```python
from build123d import *

# Parameters (mm, degrees)
SKETCH_1_R      = 1.5
EXTRUDE_1_DEPTH = 5
EXTRUDE_2_DEPTH = 10
FILLET_1_R      = 2
SKETCH_4_R      = 4.5
EXTRUDE_4_DEPTH = 110


with BuildPart() as part:
    # 草图1 → 凸台-拉伸1 (new body)
    with BuildSketch(Plane(origin=(0, 0, 0), x_dir=(1, 0, 0), z_dir=(0, 1, 0))):
        with BuildLine():
            Line((-65.462788351, 64.203800201), (-65.462788351, -59.796199799))
            ThreePointArc((-65.462788351, -59.796199799), (-64.584108695, -61.917520143), (-62.462788351, -62.796199799))
            Line((-62.462788351, -62.796199799), (158.823574937, -62.796199799))
            ThreePointArc((158.823574937, -62.796199799), (160.944895281, -61.917520143), (161.823574937, -59.796199799))
            Line((161.823574937, -59.796199799), (161.823574937, 64.203800201))
            ThreePointArc((161.823574937, 64.203800201), (160.944895281, 66.325120544), (158.823574937, 67.203800201))
            Line((158.823574937, 67.203800201), (-62.462788351, 67.203800201))
            ThreePointArc((-62.462788351, 67.203800201), (-64.584108695, 66.325120544), (-65.462788351, 64.203800201))
        make_face()
        with Locations(Location((-11.819606707, -57.796199799, 0), (0, 0, 270))):
            Circle(SKETCH_1_R, mode=Mode.SUBTRACT)
        with Locations(Location((108.180393293, -57.796199799, 0), (0, 0, 90))):
            Circle(SKETCH_1_R, mode=Mode.SUBTRACT)
        with Locations(Location((108.180393293, 62.203800201, 0), (0, 0, 270))):
            Circle(SKETCH_1_R, mode=Mode.SUBTRACT)
        with Locations(Location((-11.819606707, 62.203800201, 0), (0, 0, 90))):
            Circle(SKETCH_1_R, mode=Mode.SUBTRACT)
    extrude(amount=EXTRUDE_1_DEPTH)

    # 草图2 → 凸台-拉伸2 (add)
    with BuildSketch(Plane(origin=(0, 5, 0), x_dir=(1, 0, 0), z_dir=(0, 1, 0))):
        with BuildLine():
            Line((48.180393293, -62.796199799), (158.823574937, -62.796199799))
            ThreePointArc((158.823574937, -62.796199799), (160.944895281, -61.917520143), (161.823574937, -59.796199799))
            Line((161.823574937, -59.796199799), (161.823574937, 64.203800201))
            ThreePointArc((161.823574937, 64.203800201), (160.944895281, 66.325120544), (158.823574937, 67.203800201))
            Line((158.823574937, 67.203800201), (-62.462788351, 67.203800201))
            ThreePointArc((-62.462788351, 67.203800201), (-64.584108695, 66.325120544), (-65.462788351, 64.203800201))
            Line((-65.462788351, 64.203800201), (-65.462788351, -59.796199799))
            ThreePointArc((-65.462788351, -59.796199799), (-64.584108695, -61.917520143), (-62.462788351, -62.796199799))
            Line((-62.462788351, -62.796199799), (48.180393293, -62.796199799))
        make_face()
        Polygon((48.180393293, -52.796199799), (151.823574937, -52.796199799), (151.823574937, 57.203800201), (-55.462788351, 57.203800201), (-55.462788351, -52.796199799), align=None, mode=Mode.SUBTRACT)
    extrude(amount=EXTRUDE_2_DEPTH)

    # 圆角1
    fillet_1_edges = [part.edges().sort_by_distance(p)[0] for p in [
        (48.180393293, 15, 62.796199799),
        (160.944895281, 15, 61.917520143),
        (161.823574937, 15, -2.203800201),
        (160.944895281, 15, -66.325120544),
        (48.180393293, 15, -67.203800201),
        (-64.584108695, 15, -66.325120544),
        (-65.462788351, 15, -2.203800201),
        (-64.584108695, 15, 61.917520143),
    ]]
    fillet(fillet_1_edges, radius=FILLET_1_R)

    # 草图4 → 凸台-拉伸4 (add)
    with BuildSketch(Plane(origin=(0, 0, 52.796199799), x_dir=(-1, 0, 0), z_dir=(0, 0, -1))):
        with Locations(Location((-146.823574937, 12, 0), (0, 0, 138.189685104))):
            Circle(SKETCH_4_R)
        with Locations(Location((-136.973574937, 12, 0), (0, 0, 138.189685104))):
            Circle(SKETCH_4_R)
        with Locations(Location((-127.123574937, 12, 0), (0, 0, 138.189685104))):
            Circle(SKETCH_4_R)
        with Locations(Location((-117.273574937, 12, 0), (0, 0, 138.189685104))):
            Circle(SKETCH_4_R)
        with Locations(Location((-107.423574937, 12, 0), (0, 0, 138.189685104))):
            Circle(SKETCH_4_R)
        with Locations(Location((-97.573574937, 12, 0), (0, 0, 138.189685104))):
            Circle(SKETCH_4_R)
        with Locations(Location((-87.723574937, 12, 0), (0, 0, 138.189685104))):
            Circle(SKETCH_4_R)
        with Locations(Location((-77.873574937, 12, 0), (0, 0, 138.189685104))):
            Circle(SKETCH_4_R)
        with Locations(Location((-68.023574937, 12, 0), (0, 0, 138.189685104))):
            Circle(SKETCH_4_R)
        with Locations(Location((-58.173574937, 12, 0), (0, 0, 138.189685104))):
            Circle(SKETCH_4_R)
        with Locations(Location((-48.323574937, 12, 0), (0, 0, 138.189685104))):
            Circle(SKETCH_4_R)
        with Locations(Location((-38.473574937, 12, 0), (0, 0, 138.189685104))):
            Circle(SKETCH_4_R)
        with Locations(Location((-28.623574937, 12, 0), (0, 0, 138.189685104))):
            Circle(SKETCH_4_R)
        with Locations(Location((-18.773574937, 12, 0), (0, 0, 138.189685104))):
            Circle(SKETCH_4_R)
        with Locations(Location((-8.923574937, 12, 0), (0, 0, 138.189685104))):
            Circle(SKETCH_4_R)
        with Locations(Location((0.926425063, 12, 0), (0, 0, 138.189685104))):
            Circle(SKETCH_4_R)
        with Locations(Location((10.776425063, 12, 0), (0, 0, 138.189685104))):
            Circle(SKETCH_4_R)
        with Locations(Location((20.626425063, 12, 0), (0, 0, 138.189685104))):
            Circle(SKETCH_4_R)
        with Locations(Location((30.476425063, 12, 0), (0, 0, 138.189685104))):
            Circle(SKETCH_4_R)
        with Locations(Location((40.326425063, 12, 0), (0, 0, 138.189685104))):
            Circle(SKETCH_4_R)
        with Locations(Location((50.176425063, 12, 0), (0, 0, 138.189685104))):
            Circle(SKETCH_4_R)
    extrude(amount=EXTRUDE_4_DEPTH)


solid = part.part
```
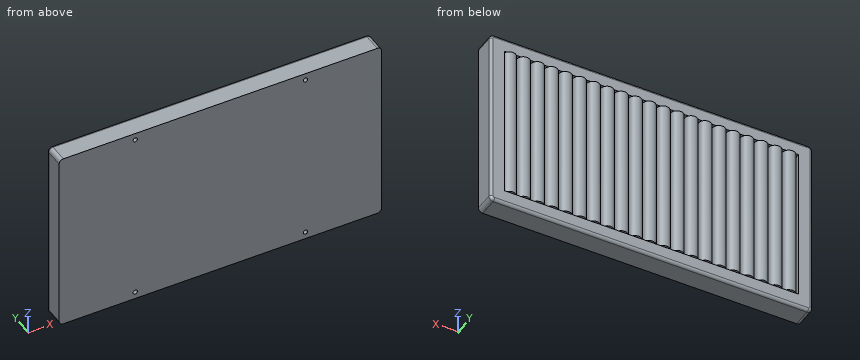
Geometry check sheet. Reference: the model listing, model coordinates, mm. Give positions to 0.01 mm unless a question says otherwise; leave off trailing zeros. Loops run counter-clockwise (first coordinate to the right, second up) from the corner with the lowest first, then second, coordinate; pieces in that order, holes last. Notation, with made-up numbers: M -24.75,8 L 24.25,8 A24 ccw 24.25,33 Z; hole C -10,62 d6. An arc over 180 degrees is marked long. Write item = value, one per line. Start each with the question number.
1. Section check B-B, the plane x = 88. Enter the section's corners in (y, z).
2. Thickness scan on probe 1 along Z at (x, y) = (-7, 7); probe 2 along X at (y, z) = (6.5, 22); probe 3 along Y at (x, z) = (107, 20). Record the ranges inside material, lowest first.
3. Section check A-A, the plane z = 7. Give the number of separate pieces and of enclosed holes in the cut face, plus the area to 3 significant figures.
4. Go/stop test with flat-tipped pins: P1, Ø1.5, axis at x = -12.5, z = 58, coming from the -Y side; P2, Ø1.2, axis at x = 39.5, y = 16, coming from the +Z side; P3, Ø1, axis at y = 14, z = -17.5, coming from the +X side. Record where each tip stops, or that it passes through.
Values follow:
q1.outline = M 0,-67.2 L 13,-67.2 A2 ccw 15,-65.2 L 15,-57.2 L 16.49,-57.2 L 16.49,52.8 L 15,52.8 L 15,60.8 A2 ccw 13,62.8 L 0,62.8 Z; hole M 5,-57.2 L 7.51,-57.2 L 7.51,52.8 L 5,52.8 Z
q2.probe_1 = -67.2 to -57.2, 52.8 to 62.8
q2.probe_2 = -65.46 to -55.46, 151.82 to 161.82
q2.probe_3 = 0 to 5, 7.52 to 16.48
q3.separate_pieces = 22
q3.enclosed_holes = 0
q3.area = 2,670 mm^2
q4.P1 = 5
q4.P2 = 52.8
q4.P3 = 161.76
